Source: CAD feature listing. Evaluate the final solid. Frame: model axes, mm. A direction names the side the tool comes from. Give positions to 0.01 mm unless a question says otherwise; leave off trailing zeros. Order: outer loops, then holes, each group sorted by start corner. A loop starts at its lowest first (then second) coordinate and runs counter-clockwise, first axis right, second up. Notation, with made-up numbers: (-0.75, 59) - (7.25, 59) arc R30 cw to (7.25, 98) - close; hole circle Ø5 at (78.25, 12). An arc over 180 degrees is marked (long way). Write each question's results on one line, items separated by ' | '. Start each with the question number.
Item 1: Set-up query: faces 1 (the flat face through (21.15, -8, 17)), 2 (the flat face through (8.9, 10.9, 31.21)), 3 (the flat face through (21.621, 1.886, 29.483)), 4 (the flat face through (14.84, 19, 17.14)), 5 (the flat face through (16.97, -17, 17)). Return all of +Z, -Z, +X, -X, +Y, -Y with unobstructed straight access to the full face (end or side cutting, diameter ignored); none if empty.
Item 2: Section A-A on z = 26. State how many separate pieces and enclosed holes the cut face has, and give its area (3 significant figures).
Item 3: Line query: line 1 along X through (y, z) = (20, 30); line 2 along Y through (x, z) = (21, 20); line 3 along Z through (x, y) = (23, -1.5). Output: solid intervals per line, ascending.
Item 4: Section B-B on x = -15.5. Output: boundary loops of the cut face in (y, z), and give its area (3 significant figures).
Item 5: Mould query, pull axis Y, two halves, no side actions, for faces 6 (the flat face through (-19, 16.97, 17)), 7 (the cylindrical face through (23.46, -2.78, 17.43)), 8 (the flat face through (16.87, 23, 17)). Classes: released by +Y, released by -Y, zero draft, split by the parting line, or undercut.
Item 6: Section D-D on x = -8. Output: boundary loops of the cut face in (y, z).
Item 7: Contact query for flat-ended pins moving along their axis: pin 1 Ø1.5 at (x, y) = (-9, 20) entering from -Z; pin 2 Ø4 at (x, z) = (-19.5, 22) entering from -Y; pin 3 Ø12 at (x, z) = (-1.5, 4.5) entering from -Y; pin 4 Ø5 at (x, y) = (17, 16.5) entering from +Z. Output: stop coordinate, or through.
Autodesk Inventor part; units mm, degrees
ref_plane "YZ Plane" through (0, 0, 0) normal (1, 0, 0) x (0, 1, 0)
ref_plane "XZ Plane" through (0, 0, 0) normal (0, 1, 0) x (-1, 0, 0)
ref_plane "XY Plane" through (0, 0, 0) normal (0, 0, 1) x (1, 0, 0)
ref_plane "Arbeitsebene1" through (0, 0, 0) normal (0, 0, 1) x (1, 0, 0)
sketch "Skizze1" plane through (0, 0, 0) normal (0, 0, 1) x (1, 0, 0)
  arc A0 (24.85, 22.85) -> (22.85, 24.85) centre (22.85, 22.85) ccw
  line L0 (22.85, 24.85) -> (-16.97, 24.85)
  line L1 (-16.97, 24.85) -> (-16.97, 21.15)
  line L2 (-16.97, 21.15) -> (16.97, 21.15)
  line L3 (16.97, 16.97) -> (16.97, 21.15)
  line L4 (21.15, 16.97) -> (16.97, 16.97)
  line L5 (21.15, 16.97) -> (21.15, -16.97)
  line L6 (21.15, -16.97) -> (24.85, -16.97)
  line L7 (24.85, -16.97) -> (24.85, 22.85)
  line L8 (23.75, 23.25) -> (23.75, 18.15)
  arc A1 (23.25, 17.65) -> (23.75, 18.15) centre (23.25, 18.15) ccw
  line L9 (23.25, 17.65) -> (20.8937, 17.65)
  arc A2 (20.5239, 17.8134) -> (20.8937, 17.65) centre (20.8937, 18.15) ccw
  line L10 (20.5239, 17.8134) -> (17.7803, 20.8273)
  arc A3 (17.65, 21.1639) -> (17.7803, 20.8273) centre (18.15, 21.1639) ccw
  line L11 (17.65, 21.1639) -> (17.65, 23.25)
  arc A4 (18.15, 23.75) -> (17.65, 23.25) centre (18.15, 23.25) ccw
  line L12 (18.15, 23.75) -> (23.25, 23.75)
  arc A5 (23.75, 23.25) -> (23.25, 23.75) centre (23.25, 23.25) ccw
  line L13 (-16.87, 24.85) -> (16.87, 24.85)
  line L14 (16.87, 24.85) -> (16.87, 21.85)
  line L15 (16.87, 21.85) -> (-16.87, 21.85)
  line L16 (-16.87, 21.85) -> (-16.87, 24.85)
  line L17 (34.79, 34.79) -> (-34.79, -34.79)
  line L18 (16.87, 21.85) -> (16.87, 16.87)
  line L19 (12.87, 21.85) -> (12.87, 12.87)
  line L20 (16.87, 16.87) -> (12.87, 12.87)
  line L21 (-16.97, 21.15) -> (-16.97, 16.97)
  line L22 (16.97, 16.97) -> (-16.97, 16.97)
  line L23 (16.97, 21.15) -> (16.97, 16.97)
  line L24 (-16.97, 21.15) -> (16.97, 21.15)
  line L25 (-16.97, 16.97) -> (-16.97, 20.75)
  line L26 (-20.75, 16.97) -> (-16.97, 20.75)
  line L27 (-20.75, 16.97) -> (-16.97, 16.97)
  line L28 (-16.87, 21.85) -> (-12.87, 21.85)
  line L29 (-12.87, 21.85) -> (-12.87, 16.97)
  line L30 (-12.87, 16.97) -> (-16.87, 16.97)
  line L31 (-16.87, 16.97) -> (-16.87, 21.85)
  line L32 (-16.87, 20.7793) -> (-20.6793, 16.97)
  line L33 (-20.6793, 16.97) -> (-16.87, 16.97)
  line L34 (-4.8794, 21.85) -> (21.15, -4.1794)
  line L35 (-7.0711, 15.5563) -> (3.471, 5.0143)
  line L36 (21.15, 2.8916) -> (2.1916, 21.85)
  line L37 (12.0208, 12.0208) -> (8.4853, 8.4853)
  line L38 (20.75, 16.97) -> (16.97, 20.75)
  line L39 (16.97, 20.6793) -> (20.6793, 16.97)
  point P0 (0, 0)
  point P1 (-12.87, 21.15)
  point P2 (12.87, 21.15)
  point P3 (2.8916, 21.15)
  point P4 (-4.1794, 21.15)
  point P5 (12.87, 16.97)
  point P6 (16.87, 21.15)
  dimension "d0" = 0.1
  dimension "d1" = 0.1
  dimension "d2" = 3
  dimension "d3" = 4
  dimension "d6" = 4
  dimension "d8" = 0
  dimension "d9" = 0.05
  dimension "d10" = 6
  dimension "d11" = 5
  dimension "d12" = 0.05
extrude "Extrusion1" add sketch "Skizze1" along normal blind 33.8 contours L14 L15 L16 L0 | L18 L2 L19 L15 | L34 L22 L36 L17 | L15 L29 L2 L31 | L19 L2 L36 L15 | L18 L22 L19 L2 | L2 L3 L22 L18 | L39 L4 L17 | L17 L3 L39 | L34 L2 L36 L22 | L15 L34 L2 L29 | L2 L29 L22 L31 | L36 L2 L34 L15 | L31 L22 L21 L32 | L21 L27 L32
mirror "Spiegeln1" about plane through (8.4853, 8.4853, 0) normal (0.7071, -0.7071, 0) of "Extrusion1"
chamfer "Fase1" distance 4 angle 45 3 edges at (12.87, 16.97, 16.9) (16.97, 12.87, 16.9) (-12.87, 16.97, 16.9)
ref_plane "Arbeitsebene2" through (21.9197, 25.629, 0) normal (0.7071, 0.7071, 0) x (-0.7071, 0.7071, 0)
sketch "Skizze2" plane through (21.9197, 25.629, 0) normal (0.7071, 0.7071, 0) x (-0.7071, 0.7071, 0)
  line L0 (-16.6229, 20.13) -> (-16.6229, 14.13)
  arc A0 (-19.6229, 14.13) -> (-16.6229, 14.13) centre (-18.1229, 14.13) ccw
  line L1 (-19.6229, 14.13) -> (-19.6229, 20.13)
  arc A1 (-16.6229, 20.13) -> (-19.6229, 20.13) centre (-18.1229, 20.13) ccw
  line L2 (0.3771, 31.21) -> (-5.6229, 31.21)
  arc A2 (-5.6229, 34.21) -> (-5.6229, 31.21) centre (-5.6229, 32.71) ccw
  line L3 (-5.6229, 34.21) -> (0.3771, 34.21)
  arc A3 (0.3771, 31.21) -> (0.3771, 34.21) centre (0.3771, 32.71) ccw
  circle A4 centre (-16.6229, 31.13) radius 3.25
  circle A5 centre (-2.6229, 17.13) radius 3.25
  circle A6 centre (11.3771, 31.13) radius 3.25
  circle A7 centre (-16.6229, 3.13) radius 3.25
  line L4 (14.3357, 42.03) -> (-19.6229, 42.03)
  line L5 (-19.6229, 42.03) -> (-19.6229, 38.4552)
  line L6 (-19.6229, 38.4552) -> (-23.9481, 34.13)
  line L7 (-23.9481, 34.13) -> (-27.5229, 34.13)
  line L8 (-27.5229, 34.13) -> (-27.5229, 0.13)
  line L9 (-27.5229, 0.13) -> (-23.9481, 0.13)
  line L10 (-23.9481, 0.13) -> (-19.6229, -4.1952)
  line L11 (-19.6229, -4.1952) -> (-19.6229, -7.77)
  line L12 (-19.6229, -7.77) -> (14.3771, -7.77)
  line L13 (14.3771, -7.77) -> (14.3771, -4.1952)
  line L14 (14.3771, -4.1952) -> (18.7023, 0.13)
  line L15 (18.7023, 0.13) -> (22.2771, 0.13)
  line L16 (22.2771, 0.13) -> (22.2771, 34.13)
  line L17 (22.2771, 34.13) -> (18.7023, 34.13)
  line L18 (18.7023, 34.13) -> (14.3357, 38.4966)
  line L19 (14.3357, 38.4966) -> (14.3357, 42.03)
  point P0 (-2.6229, 0)
hole "Bohrung1" at (13.8749, 33.6739, 31.13) at (33.6739, 13.8749, 31.13) at (33.6739, 13.8749, 3.13) direction (-0.7071, -0.7071, 0) diameter 2.8 depth 30 tip angle 118 counterbore diameter 6.5 counterbore depth 17
sketch "Skizze3" plane through (16.97, 20.6793, 0) normal (0.7071, 0.7071, 0) x (-0.7071, 0.7071, 0)
  line L0 (-16.6229, 20.13) -> (-16.6229, 14.13)
  arc A0 (-19.6229, 14.13) -> (-16.6229, 14.13) centre (-18.1229, 14.13) ccw
  line L1 (-19.6229, 14.13) -> (-19.6229, 20.13)
  arc A1 (-16.6229, 20.13) -> (-19.6229, 20.13) centre (-18.1229, 20.13) ccw
  line L2 (0.3771, 31.21) -> (-5.6229, 31.21)
  arc A2 (-5.6229, 34.21) -> (-5.6229, 31.21) centre (-5.6229, 32.71) ccw
  line L3 (-5.6229, 34.21) -> (0.3771, 34.21)
  arc A3 (0.3771, 31.21) -> (0.3771, 34.21) centre (0.3771, 32.71) ccw
  circle A4 centre (-16.6229, 31.13) radius 3.25
  circle A5 centre (-2.6229, 17.13) radius 3.25
  circle A6 centre (11.3771, 31.13) radius 3.25
  circle A7 centre (-16.6229, 3.13) radius 3.25
  line L4 (14.3357, 42.03) -> (-19.6229, 42.03)
  line L5 (-19.6229, 42.03) -> (-19.6229, 38.4552)
  line L6 (-19.6229, 38.4552) -> (-23.9481, 34.13)
  line L7 (-23.9481, 34.13) -> (-27.5229, 34.13)
  line L8 (-27.5229, 34.13) -> (-27.5229, 0.13)
  line L9 (-27.5229, 0.13) -> (-23.9481, 0.13)
  line L10 (-23.9481, 0.13) -> (-19.6229, -4.1952)
  line L11 (-19.6229, -4.1952) -> (-19.6229, -7.77)
  line L12 (-19.6229, -7.77) -> (14.3771, -7.77)
  line L13 (14.3771, -7.77) -> (14.3771, -4.1952)
  line L14 (14.3771, -4.1952) -> (18.7023, 0.13)
  line L15 (18.7023, 0.13) -> (22.2771, 0.13)
  line L16 (22.2771, 0.13) -> (22.2771, 34.13)
  line L17 (22.2771, 34.13) -> (18.7023, 34.13)
  line L18 (18.7023, 34.13) -> (14.3357, 38.4966)
  line L19 (14.3357, 38.4966) -> (14.3357, 42.03)
  point P0 (-2.6229, 0)
extrude "Extrusion2" cut sketch "Skizze3" against normal blind 33.8 contours L0 A0 L1 A1 | L2 A2 L3 A3
sketch "Skizze4" plane through (0, 0, 33.8) normal (0, 0, 1) x (1, 0, 0)
  line L0 (10.6066, 6.364) -> (6.364, 10.6066)
  line L1 (14.1421, 9.8995) -> (10.6066, 6.364)
  line L2 (9.8995, 14.1421) -> (14.1421, 9.8995)
  line L3 (9.8995, 14.1421) -> (6.364, 10.6066)
  circle A0 centre (10.3701, 10.3701) radius 1.4
  point P0 (0, 0)
  dimension "d26" = 2.8
extrude "Extrusion3" cut sketch "Skizze4" against normal blind 20 contours A0
sketch "Skizze5" plane through (24.85, -16.87, 33.8) normal (1, 0, 0) x (0, 0, -1)
  ellipse E0 centre (13.67, 19.7997) end of major axis (13.67, 21.921) minor radius 1.5 (13.67, 21.921) -> (13.67, 17.6784) ccw
  line L0 (13.67, 21.921) -> (19.67, 21.921)
  ellipse E1 centre (19.67, 19.7997) end of major axis (19.67, 17.6784) minor radius 1.5 (19.67, 17.6784) -> (19.67, 21.921) ccw
  line L1 (19.67, 17.6784) -> (13.67, 17.6784)
  ellipse E2 centre (2.67, 21.921) end of major axis (2.67, 26.5172) minor radius 3.25 (0, 19.3005) -> (0, 24.5415) ccw
  line L2 (0, 19.3005) -> (0, 0)
  line L3 (33.8, 0) -> (0, 0)
  line L4 (33.8, 20.6836) -> (33.8, 0)
  ellipse E3 centre (30.67, 21.921) end of major axis (30.67, 26.5172) minor radius 3.25 (33.8, 23.1584) -> (33.8, 20.6836) ccw
  line L5 (33.8, 33.74) -> (33.8, 23.1584)
  line L6 (33.8, 33.74) -> (0, 33.74)
  line L7 (0, 33.74) -> (0, 24.5415)
  line L8 (19.67, 15.4558) -> (13.67, 15.4558)
  circle A0 centre (16.67, 15.4558) radius 1.4
  point P0 (33.8, 16.87)
  dimension "d29" = 2.8
extrude "Extrusion4" cut sketch "Skizze5" against normal blind 20 contours A0 L8 | L8 A0
properties part number "20_Cube_Insert_Kinematic_Mirror_45_pro_v3"
Evaluation:
1) face 1: +Z, -Z, -X | face 2: +Z | face 3: none | face 4: +Z, -Z | face 5: +Z, -Z, -X, -Y
2) separate pieces: 1 | enclosed holes: 2 | area: 463 mm^2
3) line 1: x = -17.65 to -13.84, -3.03 to -0.97, 1.37 to 3.51, 13.84 to 17.65 | line 2: y = -16.87 to -12.87, -4.03 to -3.04, 1.2 to 3.04, 12.87 to 16.97 | line 3: z = 0 to 15.73, 18.53 to 33.8
4) outline: (18.34, 0) - (24.85, 0) - (24.85, 33.8) - (18.34, 33.8) - close | area: 220 mm^2
5) face 6: released by -Y | face 7: undercut | face 8: zero draft
6) outline: (21.15, 0) - (24.85, 0) - (24.85, 33.8) - (21.15, 33.8) - close
7) pin 1: passes through | pin 2: stops at y = 16.97 | pin 3: stops at y = 12.47 | pin 4: stops at z = 31.21
